Could you check a few things on this drawing? It's one solid part, dimensions in mm from its lowest x, y, z. A direction names the side the tool comes from. Round coordinates to 2 decimals unless told otherwise and drop trailing zeros. Write each loop counter-clockwise with the first axis right and the second up, starting at its lowest first coordinate (ties: lowest second). Pieces come first, ordered by that corner, then holes. Notation, with made-up numbers: (48, 10.25) -> (52, 10.25) arc R10 cw to (52, 20.25) -> close; hole circle Ø5 at (16.25, 17). An arc over 180 degrees is marked (long way). Put each result on its own line as item: value. Start each with the question number.
1) Which directions (+Z, -Z, +X, -X, +Y, -Y) give clear straight access to the entire face, cutting with the end or side of a thin tool? Please do the marked faces 1 and 2.
2) I want a section at D-D, the plane z = 4. List the corners of the cut face in (x, y) for me.
3) Will these pins go through, and if not, where does the flat tip stop? P1, Ø2.5, axis at y = 12, z = 4, coming from the +X side; P2, Ø2, axis at x = 14.5, y = 4.5, coming from the -Z side; P3, Ø4, axis at y = 18.5, z = 13.5, coming from the +X side.
4) I want a section at B-B, the plane y = 12. List the corners of the cut face in (x, z) for me, then the cut area to 3 significant figures.
5) I want a section at A-A, the plane x = 12. List the corners of the cut face in (y, z) for me.
6) I want a section at C-C, the plane z = 36. List the corners of the cut face in (x, y) for me, then the cut area to 3 significant figures.
7) If I drill on line 1 along Z through (x, y) = (11, 12); line 2 along Z through (x, y) = (1.5, 11.25); line 3 along X through (y, z) = (12, 19.5), over which ranges is the centre line in solid material (lowest first)? Write a range as [from, to].
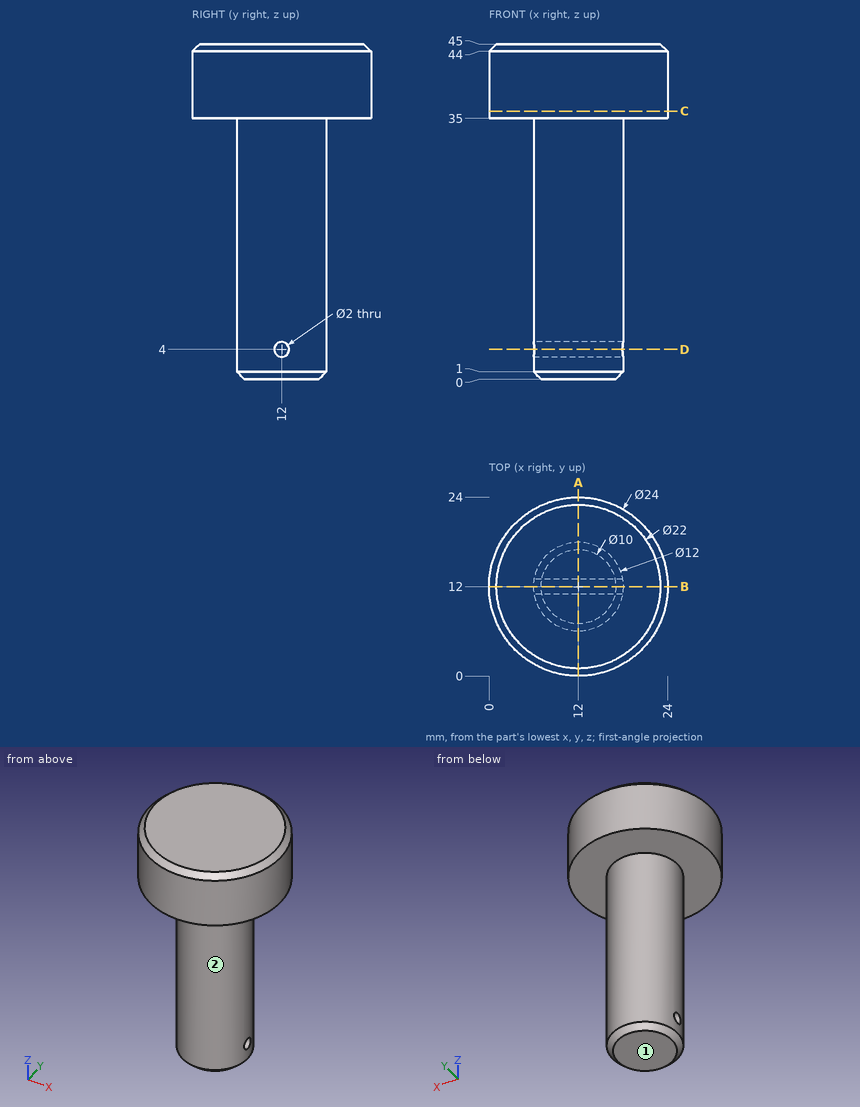
Findings:
1. face 1: -Z, +X, -X, +Y, -Y
1. face 2: -Z
2. outline: (6.08, 11) arc R6 ccw to (17.92, 11) -> close; (6.08, 13) -> (17.92, 13) arc R6 ccw to start
3. P1: stops at x = 18
3. P2: stops at z = 35
3. P3: stops at x = 15.97
4. outline: (0, 35) -> (6, 35) -> (6, 5) -> (18, 5) -> (18, 35) -> (24, 35) -> (24, 44) -> (23, 45) -> (1, 45) -> (0, 44) -> close; (6, 1) -> (7, 0) -> (17, 0) -> (18, 1) -> (18, 3) -> (6, 3) -> close
4. area: 634 mm2
5. outline: (0, 35) -> (6, 35) -> (6, 1) -> (7, 0) -> (17, 0) -> (18, 1) -> (18, 35) -> (24, 35) -> (24, 44) -> (23, 45) -> (1, 45) -> (0, 44) -> close; hole circle Ø2 at (12, 4)
6. outline: circle Ø24 at (12, 12)
6. area: 452 mm2
7. line 1: z = [0, 3], [5, 45]
7. line 2: z = [35, 45]
7. line 3: x = [6, 18]
